Geometry check sheet. Reference: drawing and pictorial views, mm from the part's lowest x, y, z. A direction names the side the tool comes from. Coordinates: 2 decimals unless noted, no trailing zeros. Write each loop counter-clockwise with the first axis right and the second up, starting at its lowest first coordinate (ties: lowest second). Pieces come first, ordered by that corner, then holes. Notation, with made-up numbers: (78.5, 68.25) - (112.5, 68.25) arc R20 ccw to (112.5, 77.25) - close; hole circle Ø11 at (-8.75, 47.25). An arc over 180 degrees is marked (long way). Use one line per item in the form item = value. Start each with the question number.
(1) Material ranges on line 1 (Y direction, x = 10.5, z = 19.5); line 2 (Z direction, x = 9.75, y = 3.5); line 3 (Y direction, x = 6, z = 38), recorded low to high. Write a range as [from, to].
(2) Tool access check on the marked faces 1 and 2. Record the directions out of +Z, -Z, +X, -X, +Y, -Y that give a thin tool (end or side, any length) a straight path to the whole face; none if there is none.
(3) Sectioned sample at A-A (z = 19.5). Record the cut outline in (x, y), and give its area (3 significant figures).
(4) Gauge pin test, flat ends, axial feed: pin 1 Ø3 at (x, y) = (8.5, 16) entering from -Z; pin 2 Ø6 at (x, z) = (12.5, 10.5) entering from -Y; pin 3 Ø1.4 at (x, y) = (12.5, 0.5) entering from +Z. Record the tip position at first contact, or that the pin passes through.
(5) Sectioned sample at C-C (x = 11.5). Record the cut outline in (y, z), and give its area (3 significant figures).
(6) Sectioned sample at B-B (y = 3.5). Record the cut outline in (x, z).
(7) Mould release check, pull along X, two halves, no side actions. Record for the marked faces 3, 4 and 5: released by +X, released by -X, zero draft, split by the parting line, or undercut.
(8) Sectioned sample at D-D (y = 14). Record the cut outline in (x, z), and give its area (3 significant figures).
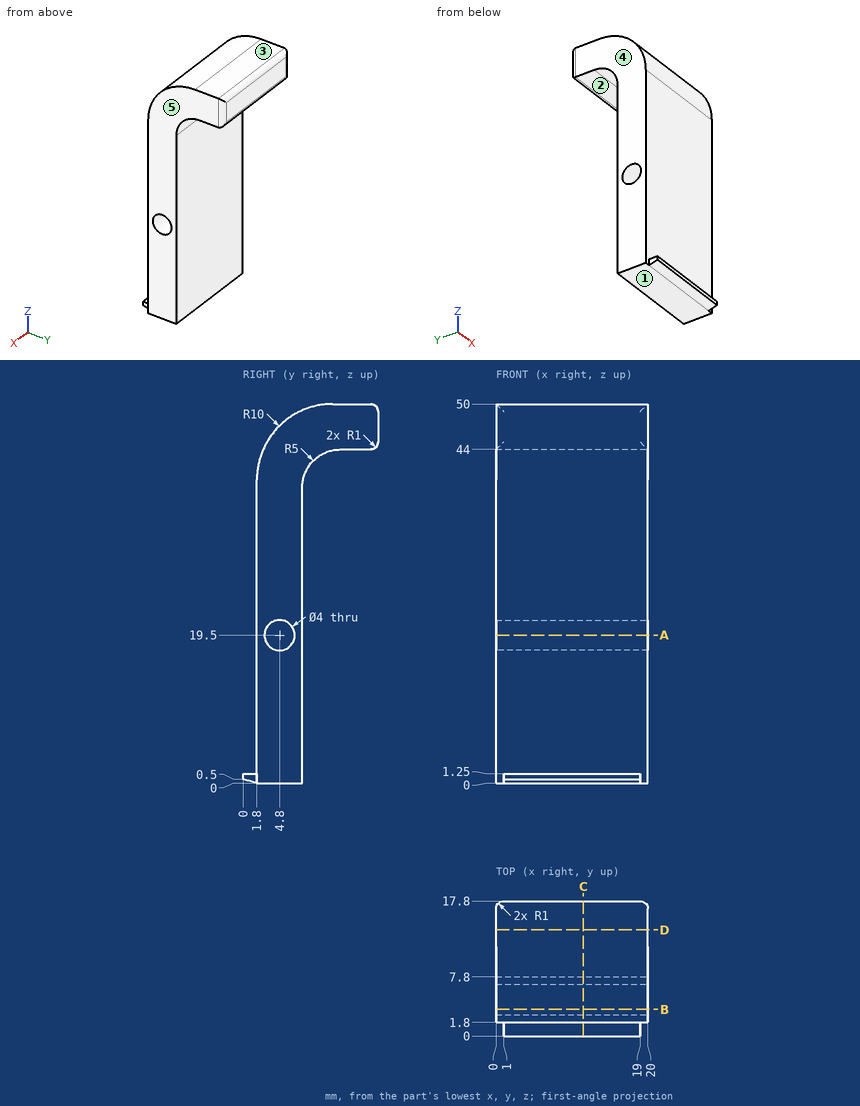
Answers below:
q1.line_1 = [1.8, 2.8], [6.8, 7.8]
q1.line_2 = [0, 17.98], [21.02, 45.58]
q1.line_3 = [1.8, 7.8]
q2.face_1 = -Z, +X, -X, +Y, -Y
q2.face_2 = -Z, +X, -X, +Y
q3.outline = (0, 1.8) - (20, 1.8) - (20, 2.8) - (0, 2.8) - close; (0, 6.8) - (20, 6.8) - (20, 7.8) - (0, 7.8) - close
q3.area = 40.0 mm2
q4.pin_1 = 44
q4.pin_2 = 1.8
q4.pin_3 = 1.25
q5.outline = (0, 0.5) - (1.8, 0) - (7.8, 0) - (7.8, 39) arc R5 cw to (12.8, 44) - (16.8, 44) arc R1 ccw to (17.8, 45) - (17.8, 49) arc R1 ccw to (16.8, 50) - (11.8, 50) arc R10 ccw to (1.8, 40) - (1.8, 1.25) - (0, 1.25) - close; hole circle Ø4 at (4.8, 19.5)
q5.area = 333 mm2
q6.outline = (0, 0) - (20, 0) - (20, 17.98) - (0, 17.98) - close; (0, 21.02) - (20, 21.02) - (20, 45.58) - (0, 45.58) - close
q7.face_3 = zero draft
q7.face_4 = released by -X
q7.face_5 = released by +X
q8.outline = (0, 44) - (20, 44) - (20, 50) - (0, 50) - close
q8.area = 120 mm2
